Verification items for the finished model (mm, model axes). A direction names the side the tool comes from. Round coordinates to 2 decimals unless told otherwise and drop trailing zeros. Order: outer loops, then holes, each group sorted by start corner. A loop starts at its lowest first (then second) coordinate and runs counter-clockwise, first axis right, second up. Notation, with made-up numbers: (21, 22) -> (48, 22) arc R17 cw to (48, 26) -> close; hole circle Ø11 at (68, -17). An arc over 180 degrees is marked (long way). Put each result on its own line as item: value.
```python
from build123d import *

# Parameters (mm, degrees)
F1_DEPTH = 25


with BuildPart() as f1:
    # F0 (on Top) → F1 (new body)
    with BuildSketch(Plane.XY):
        with BuildLine():
            ThreePointArc((1.863135, 8.365539), (9.863135, 0.365539), (1.863135, -7.634461))
            Line((1.863135, -7.634461), (-5.573545, -7.634461))
            Line((-5.573545, -7.634461), (-5.573545, -21.884736))
            Line((-5.573545, -21.884736), (24.369754, -20.425071))
            Line((24.369754, -20.425071), (24.369754, 21.156149))
            Line((24.369754, 21.156149), (-5.573545, 22.615814))
            Line((-5.573545, 22.615814), (-5.573545, 8.365539))
            Line((-5.573545, 8.365539), (1.863135, 8.365539))
        make_face()
    extrude(amount=F1_DEPTH)


solid = f1.part
```
Item 1: Tool access check on faces 1 (the face through (-2, 8.366, 12)), 2 (the face through (-5.574, 16, 12)). Record the directions out of +Z, -Z, +X, -X, +Y, -Y that give a thin tool (end or side, any length) a straight path to the whole face; none if there is none.
Geometry check:
face 1: +Z, -Z, -X
face 2: +Z, -Z, -X, +Y, -Y
Item 2: Release check for a two-part mould opening along Y. For faces 3 (the face through (-5.574, -15, 12)), 4 (the face through (9.608, 21.876, 12.325)), 5 (the face through (9.86, 0.54, 12.32)) record: pulls with the +Y half, pulls with the -Y half, needs draft (parallel to the pull), parting line crosses it, or undercut.
Geometry check:
face 3: needs draft
face 4: pulls with the +Y half
face 5: undercut
Item 3: Sectioned sample at C-C, the plane x = -2. Record the boundary of the cut face in (y, z).
Geometry check:
outline: (-21.71, 0) -> (-7.63, 0) -> (-7.63, 25) -> (-21.71, 25) -> close; (8.37, 0) -> (22.44, 0) -> (22.44, 25) -> (8.37, 25) -> close
Item 4: Sectioned sample at A-A, the plane x = 7.25. Record the boundary of the cut face in (y, z).
Geometry check:
outline: (-21.26, 0) -> (-5.55, 0) -> (-5.55, 25) -> (-21.26, 25) -> close; (6.28, 0) -> (21.99, 0) -> (21.99, 25) -> (6.28, 25) -> close
Item 5: Depth check by flat-ended pin: pin 1 Ø3.5 at (x, z) = (-1.5, 8.5) entering from -Y; pin 2 Ø1.5 at (x, z) = (16.5, 12.5) entering from -Y; pin 3 Ø6 at (x, z) = (-1.5, 13.5) entering from +Y. Enter the tip coordinate at first touch or a pass-through.
Geometry check:
pin 1: y = -21.77
pin 2: y = -20.85
pin 3: y = 22.56
Item 6: Material ranges on line 1 along Y through (x, z) = (6.75, 16); line 2 along Y through (x, z) = (-3, 6); line 3 along X through (y, z) = (0.5, 13.75), recorded low to high.
Geometry check:
line 1: -21.28 to -5.97, 6.7 to 22.02
line 2: -21.76 to -7.63, 8.37 to 22.49
line 3: 9.86 to 24.37
Item 7: Sectioned sample at B-B, the plane z = 17. Record the boundary of the cut face in (x, y), then the cut area to 3 significant figures.
Geometry check:
outline: (-5.57, -21.88) -> (24.37, -20.43) -> (24.37, 21.16) -> (-5.57, 22.62) -> (-5.57, 8.37) -> (1.86, 8.37) arc R8 cw to (1.86, -7.63) -> (-5.57, -7.63) -> close
area: 1,070 mm2
Item 8: Sectioned sample at D-D, the plane y = -6. Record the boundary of the cut face in (x, z), then the cut area to 3 significant figures.
Geometry check:
outline: (6.71, 0) -> (24.37, 0) -> (24.37, 25) -> (6.71, 25) -> close
area: 442 mm2
